The listing builds one solid part. Answer for the finished solid, in the listing's coordinates (mm). Face numbers are marked on the shaded views. A direction names the side the tool comes from. Give positions to 0.01 mm unless a question says otherwise; leave off trailing zeros. Write each loop counter-clockwise with the first axis right and the second up, starting at its lowest first coordinate (ties: lowest second). Pieces come first, ordered by that corner, then holes. Notation, with made-up numbers: (-24, -39) - (15, -39) arc R26 ccw to (15, -20) - close; hole circle Ø9 at (18.25, 58). An arc over 180 degrees is marked (long way). One line per item, written item: value. Start each with the question number.
from build123d import *

# Parameters (mm, degrees)
SKETCH1_R           = 50.8
BOSS_EXTRUDE1_DEPTH = 33.274
SKETCH3_R           = 44.45
BOSS_EXTRUDE2_DEPTH = 19.05
SKETCH5_R           = 25.4
CUT_EXTRUDE1_DEPTH  = 53.324


with BuildPart() as part:
    # Sketch1 → Boss-Extrude1 (new body)
    with BuildSketch(Plane.XY):
        Circle(SKETCH1_R)
    extrude(amount=BOSS_EXTRUDE1_DEPTH)

    # Sketch3 → Boss-Extrude2 (add)
    with BuildSketch(Plane.XY.offset(33.274)):
        Circle(SKETCH3_R)
    extrude(amount=BOSS_EXTRUDE2_DEPTH)

    # Sketch5 → Cut-Extrude1 (cut, through all)
    with BuildSketch(Plane.XY):
        Circle(SKETCH5_R)
    extrude(amount=CUT_EXTRUDE1_DEPTH, mode=Mode.SUBTRACT)


solid = part.part
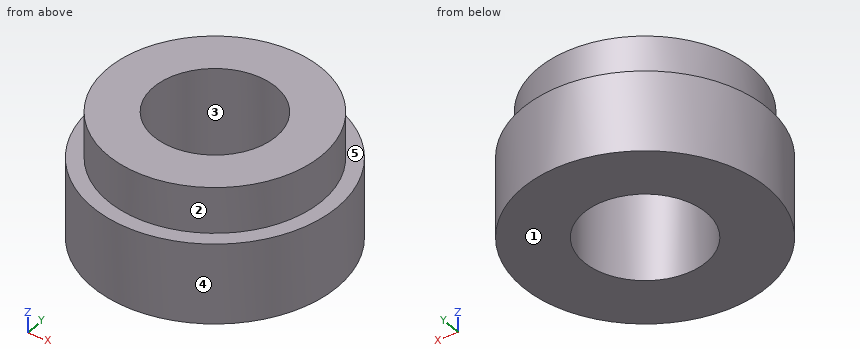
Item 1: Find section C-C on z = 12. Determine the outline of the cut face in (x, y), plus the area to 3 significant figures.
Item 2: Each of these flat-tipped pins is pushed along its axis until it touches: pin 1 Ø12 at (y, z) = (23, 27.5) entering from -X; pin 2 Ø5 at (x, z) = (26, 8) entering from -Y; pin 3 Ø4 at (x, z) = (5, 6.5) entering from +Y. Where does it stop, or does it pass through?
Item 3: Find section D-D on y = -37.5. Determine the outline of the cut face in (x, z), plus the area to 3 significant figures.
Item 4: Straight lines are drawn through the part: line 1 along Y through (x, z) = (0, 20); line 2 along Y through (x, z) = (0, 38); line 3 along X through (y, z) = (-11, 38.5). For each, find the intervals that lie inside material, in ascending order.
Item 5: Find section A-A on x = 0. Determine the outline of the cut face in (y, z), plus the area to 3 significant figures.
Item 6: For the marked faces 4 and 5, determine the directions among +Z, -Z, +X, -X, +Y, -Y from which every point of the face is accessible in a straight line to the end or side of a thin tool.
Item 7: The mould has two halves that part along Y. Classify the marked faces 1, 2 and 3: +Y half, -Y half, draft (parallel to the pull), parting line (faces both ways), or undercut.
Values:
1. outline: circle Ø101.6 at (0, 0); hole circle Ø50.8 at (0, 0)
1. area: 6,080 mm^2
2. pin 1: x = -47.87
2. pin 2: y = -45.04
2. pin 3: y = 50.71
3. outline: (-34.27, 0) - (34.27, 0) - (34.27, 33.27) - (23.87, 33.27) - (23.87, 52.32) - (-23.87, 52.32) - (-23.87, 33.27) - (-34.27, 33.27) - close
3. area: 3,190 mm^2
4. line 1: -50.8 to -25.4, 25.4 to 50.8
4. line 2: -44.45 to -25.4, 25.4 to 44.45
4. line 3: -43.07 to -22.89, 22.89 to 43.07
5. outline: (-50.8, 0) - (-25.4, 0) - (-25.4, 52.32) - (-44.45, 52.32) - (-44.45, 33.27) - (-50.8, 33.27) - close; (25.4, 0) - (50.8, 0) - (50.8, 33.27) - (44.45, 33.27) - (44.45, 52.32) - (25.4, 52.32) - close
5. area: 2,420 mm^2
6. face 4: +Z, -Z
6. face 5: +Z
7. face 1: draft
7. face 2: parting line
7. face 3: undercut
